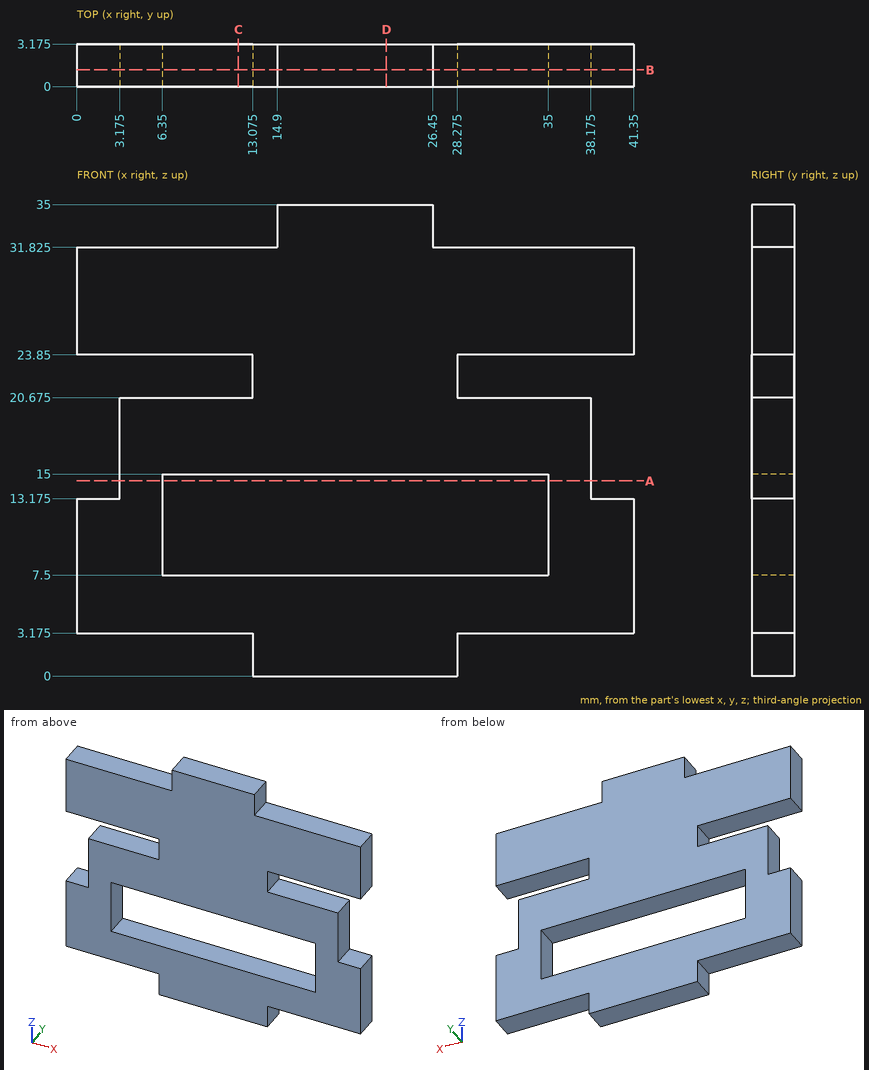
Here's the drawing with two shaded views (mm, measured from the low corner). I have some questions. Coordinates: 2 decimals unless noted, no trailing zeros. Write each loop counter-clockwise with the first axis right and the second up, starting at its lowest first coordinate (ties: lowest second). Pieces come first, ordered by that corner, then holes. Notation, with made-up numbers: M 7.25,27 L 58.25,27 A9 cw 58.25,31 Z; hole C 69,66.5 d5. An arc over 180 degrees is marked long. Answer as CSV lines item,"result".
Item 1: Imagine slicing it at A-A on z = 14.5. List the corners of the cut face in (x, y) for me (3 decimals).
Geometry results:
outline,"M 3.175,0 L 6.35,0 L 6.35,3.175 L 3.175,3.175 Z; M 35,0 L 38.175,0 L 38.175,3.175 L 35,3.175 Z"
Item 2: Imagine slicing it at D-D on x = 23. List the corners of the cut face in (y, z) for me (3 decimals), plus the area to 3 significant figures.
Geometry results:
outline,"M 0,0 L 3.175,0 L 3.175,7.5 L 0,7.5 Z; M 0,15 L 3.175,15 L 3.175,35 L 0,35 Z"
area,"87.3 mm2"
Item 3: Imagine slicing it at B-B on y = 1.25. List the corners of the cut face in (x, z) for me (3 decimals).
Geometry results:
outline,"M 0,3.175 L 13.075,3.175 L 13.075,0 L 28.275,0 L 28.275,3.175 L 41.35,3.175 L 41.35,13.175 L 38.175,13.175 L 38.175,20.675 L 28.275,20.675 L 28.275,23.85 L 41.35,23.85 L 41.35,31.825 L 26.45,31.825 L 26.45,35 L 14.9,35 L 14.9,31.825 L 0,31.825 L 0,23.85 L 13.075,23.85 L 13.075,20.675 L 3.175,20.675 L 3.175,13.175 L 0,13.175 Z; hole M 6.35,7.5 L 35,7.5 L 35,15 L 6.35,15 Z"
Item 4: I'm going to push flat-ended pins straight in: P1, Ø1, axis at x = 8.5, y = 1, coming from the -Z side (3 decimals); P2, Ø10, axis at x = 32, z = 11.5, coming from the +Y side (3 decimals); P3, Ø1, axis at x = 1.5, y = 2, coming from the +Z side (3 decimals); P4, Ø1.6, axis at y = 1, z = 2, coming from the +X side (3 decimals). Where does each tip first touch, or does it pass through?
Geometry results:
P1,"stops at z = 3.175"
P2,"stops at y = 3.175"
P3,"stops at z = 31.825"
P4,"stops at x = 28.275"
Item 5: Imagine slicing it at C-C on x = 12. List the corners of the cut face in (y, z) for me (3 decimals), plus the area to 3 significant figures.
Geometry results:
outline,"M 0,3.175 L 3.175,3.175 L 3.175,7.5 L 0,7.5 Z; M 0,15 L 3.175,15 L 3.175,20.675 L 0,20.675 Z; M 0,23.85 L 3.175,23.85 L 3.175,31.825 L 0,31.825 Z"
area,"57.1 mm2"
Item 6: Please list where these lines run through material, in increasing order: line 1 along Z through (x, y) = (16, 2.85); line 2 along X through (y, z) = (0.5, 13.5) (3 decimals); line 3 along Z through (x, y) = (4.5, 2.8) (3 decimals).
Geometry results:
line 1,"z = 0 to 7.5, 15 to 35"
line 2,"x = 3.175 to 6.35, 35 to 38.175"
line 3,"z = 3.175 to 20.675, 23.85 to 31.825"
